The model under review builds one solid part; all positions refer to its coordinate system, in mm. A direction names the side the tool comes from. Give positions to 0.01 mm unless a question says otherwise; leave off trailing zeros. Write each loop counter-clockwise with the first axis right and the second up, starting at its lowest first coordinate (ties: lowest second). Pieces come first, ordered by that corner, then holes. Notation, with made-up numbers: (28, 56.25) - (54, 56.25) arc R20 ccw to (54, 64.25) - close; hole circle Ø4 at (-25.75, 0.25). An arc over 180 degrees is marked (long way). Write item = value, one per line.
```python
from build123d import *

# Parameters (mm, degrees)
F0_W         = 60
F0_H         = 20
F1_DEPTH     = 5
F2_W         = 60
F2_H         = 6
F3_DEPTH     = 5
F4_R         = 2.75
F5_DEPTH     = 25
F6_W         = 11.2
F6_H         = 6
F7_DEPTH     = 5
F8_R         = 2.6
F9_DEPTH     = 5
F10_R        = 2.6
F11_DEPTH    = 4
F12_R        = 1
F13_C1_SIZE2 = 0.5
F13_C1_SIZE  = 0.2886751346
F13_C2_SIZE2 = 0.5
F13_C2_SIZE  = 0.2886751346


# Not quite as in the source:
# - a feature names something its author has since deleted; it is built from what else it names


with BuildPart() as f1:
    # F0 (on Top) → F1 (new body)
    with BuildSketch(Plane.XY):
        with Locations((30, 0)):
            Rectangle(F0_W, F0_H)
    extrude(amount=F1_DEPTH)

    # F2 (on face) → F3 (join)
    with BuildSketch(Plane.XY.offset(5)):
        with Locations((30, 0)):
            Rectangle(F2_W, F2_H)
    extrude(amount=F3_DEPTH)

    # F4 (on face) → F5 (cut)
    with BuildSketch(Plane.XY.offset(10)):
        with Locations((30, 0)):
            Circle(F4_R)
        with Locations((10, 0)):
            Circle(F4_R)
    extrude(amount=-F5_DEPTH, mode=Mode.SUBTRACT)

    # F6 (on face) → F7 (cut, through all)
    with BuildSketch(Plane.XY.offset(10)):
        with Locations((48.35, 0)):
            Rectangle(F6_W, F6_H)
    extrude(amount=-F7_DEPTH, mode=Mode.SUBTRACT)

    # F8 (on face) → F9 (cut, through all)
    with BuildSketch(Plane.XY.offset(5)):
        with Locations((48.35, 0)):
            Circle(F8_R)
    extrude(amount=-F9_DEPTH, mode=Mode.SUBTRACT)

    # F10 (on face) → F11 (join)
    with BuildSketch(Plane(origin=(0, 0, 0), x_dir=(0, -1, 0), z_dir=(-1, 0, 0))):
        Polygon((-10, 25), (-10, 5), (-3, 5), (-3, 10), (3, 10), (3, 5), (10, 5), (10, 25), align=None)
        with Locations((0, 15)):
            Circle(F10_R, mode=Mode.SUBTRACT)
        Polygon((-10, 5), (-10, 0), (10, 0), (10, 5), (3, 5), (3, 10), (-3, 10), (-3, 5), align=None)
    extrude(amount=F11_DEPTH)

    # F12
    f12_edges = [f1.edges().sort_by_distance(p)[0] for p in [
        (-2, -10, 25),
        (-2, 10, 25),
        (28, -10, 0),
        (28, 10, 0),
    ]]
    fillet(f12_edges, radius=F12_R)

    # F13: chamfer of 0.5 x 0.2886751346 on 2 edges, made by hand

    # F13_c1
    f13_c1_edges = [f1.edges().sort_by_distance(p)[0] for p in [
        (7.25, 0, 0),
    ]]
    f13_c1_side = f1.faces().sort_by_distance((7.2442264973, 0, 0))[0]
    chamfer(f13_c1_edges, length=F13_C1_SIZE, length2=F13_C1_SIZE2, reference=f13_c1_side)

    # F13_c2
    f13_c2_edges = [f1.edges().sort_by_distance(p)[0] for p in [
        (27.25, 0, 0),
    ]]
    f13_c2_side = f1.faces().sort_by_distance((27.2442264973, 0, 0))[0]
    chamfer(f13_c2_edges, length=F13_C2_SIZE, length2=F13_C2_SIZE2, reference=f13_c2_side)


solid = f1.part
```
1. Insertion check: P1, Ø3, axis at y = -8, z = 22.5, coming from the +X side; P2, Ø3, axis at x = 19.5, y = 1, coming from the +Z side; P3, Ø4, axis at x = 48.35, y = 0, coming from the +Z side; P4, Ø4, axis at x = 26.5, z = 8, coming from the +Y side. Each pin has a flat end and moves straight along its axis. Give the tip position at first contact, or say it passes through.
Findings below:
P1 = 0
P2 = 10
P3 = through
P4 = 3
2. Take a section at B-B on x = 48.35. Give the boundary of the cut face in (y, z).
Findings below:
outline = (-10, 1) arc R1 ccw to (-9, 0) - (-2.6, 0) - (-2.6, 5) - (-10, 5) - close; (2.6, 0) - (9, 0) arc R1 ccw to (10, 1) - (10, 5) - (2.6, 5) - close
3. Take a section at D-D on y = -5.75. Give the boundary of the cut face in (x, z), and give its area (3 significant figures).
Findings below:
outline = (-4, 0) - (60, 0) - (60, 5) - (0, 5) - (0, 25) - (-4, 25) - close
area = 400 mm²
4. Take a section at C-C on y = 0. Count the separate pieces of the cut face and the enclosed holes in it, and give its area (3 significant figures).
Findings below:
separate_pieces = 5
enclosed_holes = 0
area = 487 mm²
5. For line 1 (Y direction, x = 10, z = 2.5); line 2 (Y direction, x = 48.35, z = 3.4); line 3 (X direction, y = -0.75, z = 1), list the stretches that pass through material, from the lowest coordinate up. Write a range as from..to.
Findings below:
line_1 = -10..-2.75, 2.75..10
line_2 = -10..-2.6, 2.6..10
line_3 = -4..7.35, 12.65..27.35, 32.65..45.86, 50.84..60
6. Take a section at A-A on z = 16. Give the boundary of the cut face in (x, y), and give its area (3 significant figures).
Findings below:
outline = (-4, -10) - (0, -10) - (0, -2.4) - (-4, -2.4) - close; (-4, 2.4) - (0, 2.4) - (0, 10) - (-4, 10) - close
area = 60.8 mm²
7. Draft analysis for pull direction X (two halves, no side actions). For faces 1 (the flat face through (21, 0, 10)), 2 (the flat face through (60, 0, 4)), 3 (the flat face through (42.75, 0, 8)), state which applies: +X half, -X half, draft (parallel to the pull), parting line (faces both ways), or undercut.
Findings below:
face_1 = draft
face_2 = +X half
face_3 = undercut
8. Machinability: for faces 4 (the flat face through (57, 0, 10)), 5 (the flat face through (57, -3, 7)), 6 (the flat face through (21, 3, 7)), which of the approach directions +Z, -Z, +X, -X, +Y, -Y give a long, thin tool a straight path to every point of the face, cutting with its end or side? Answer none if there is none.
Findings below:
face_4 = +Z, +X, +Y, -Y
face_5 = +Z, +X, -Y
face_6 = +Z, +X, +Y
